Work out the finished part from the listing and answer in its coordinate system (mm). A direction names the side the tool comes from. Coordinates: 2 decimals unless noted, no trailing zeros. Loops run counter-clockwise (first coordinate to the right, second up) from the corner with the lowest first, then second, coordinate; pieces in that order, holes last. Notation, with made-up numbers: M 55,46.5 L 82,46.5 A14 cw 82,58.5 Z; hole C 6,34 d3. An arc over 180 degrees is marked long. Write each question's results on one line, items separated by ' | '.
```python
from build123d import *

# Parameters (mm, degrees)
F0_R     = 4.2
F0_W     = 2
F0_H     = 4.4
F0_W_2   = 1
F1_DEPTH = 16.4
F2_DEPTH = 6.2
F3_DEPTH = 14
F4_R     = 0.5


with BuildPart() as f1:
    # F0 (on Top) → F1 (new body)
    with BuildSketch(Plane.XY):
        Circle(F0_R)
        Polygon((-2.5, -2.2), (-2.5, 2.2), (-0.5, 2.2), (0.5, 2.2), (2.5, 2.2), (2.5, -2.2), (0.5, -2.2), (-0.5, -2.2), align=None, mode=Mode.SUBTRACT)
        with Locations((-1.5, 0)):
            Rectangle(F0_W, F0_H)
        with Locations((1.5, 0)):
            Rectangle(F0_W, F0_H)
        Rectangle(F0_W_2, F0_H)
    extrude(amount=F1_DEPTH)

    # F0 (on Top) → F2 (cut)
    with BuildSketch(Plane.XY):
        with Locations((1.5, 0)):
            Rectangle(F0_W, F0_H)
        with Locations((-1.5, 0)):
            Rectangle(F0_W, F0_H)
        Rectangle(F0_W_2, F0_H)
    extrude(amount=F2_DEPTH, mode=Mode.SUBTRACT)

    # F0 (on Top) → F3 (cut)
    with BuildSketch(Plane.XY):
        with Locations((1.5, 0)):
            Rectangle(F0_W, F0_H)
        with Locations((-1.5, 0)):
            Rectangle(F0_W, F0_H)
    extrude(amount=F3_DEPTH, mode=Mode.SUBTRACT)

    # F4
    f4_edges = [f1.edges().sort_by_distance(p)[0] for p in [
        (-4.2, 0, 16.4),
    ]]
    fillet(f4_edges, radius=F4_R)


solid = f1.part
```
1) Find section D-D, the plane x = 0. Give the vertices of the cut face in (y, z).
Check result:
outline: M -4.2,0 L -2.2,0 L -2.2,6.2 L 2.2,6.2 L 2.2,0 L 4.2,0 L 4.2,15.9 A0.5 ccw 3.7,16.4 L -3.7,16.4 A0.5 ccw -4.2,15.9 Z
2) Find section A-A, the plane z = 6.75. Give the vertices of the cut face in (x, y).
Check result:
outline: C 0,0 d8.4; hole M -2.5,-2.2 L -0.5,-2.2 L -0.5,2.2 L -2.5,2.2 Z; hole M 0.5,-2.2 L 2.5,-2.2 L 2.5,2.2 L 0.5,2.2 Z
3) Straight lines are drawn through the part: probe 1 along X at (y, z) = (-2, 13.75); probe 2 along X at (y, z) = (-1, 10.25); probe 3 along X at (y, z) = (1.25, 4.75). For each, find the intervals that lie inside material, in ascending order. Write a range as [from, to].
Check result:
probe 1: [-3.69, -2.5], [-0.5, 0.5], [2.5, 3.69] | probe 2: [-4.08, -2.5], [-0.5, 0.5], [2.5, 4.08] | probe 3: [-4.01, -2.5], [2.5, 4.01]
4) Given pin 1 Ø2 at (x, y) = (2, 0.5) entering from -Z; pin 2 Ø1.5 at (x, z) = (-3, 9.5) entering from -Y; pin 3 Ø3 at (x, z) = (2.5, 9.5) entering from -Y; pin 4 Ø1.5 at (y, z) = (2.5, 12) entering from -X, each flat-ended and moving along its own axis, determine where each tip first touches the part or whether it passes through.
Check result:
pin 1: z = 0 | pin 2: y = -3.55 | pin 3: y = -4.08 | pin 4: x = -3.82
5) Which of the six approach directions +Z, -Z, +X, -X, +Y, -Y give full straight-line access (tool end or side, diameter ignored) to faces 1 (the face through (2.5, 0, 7)), 2 (the face through (3, 0, 0))?
Check result:
face 1: -Z | face 2: -Z, +X, -X, +Y, -Y
6) Find section B-B, the plane z = 4.5. Give the vertices of the cut face in (x, y).
Check result:
outline: C 0,0 d8.4; hole M -2.5,-2.2 L 2.5,-2.2 L 2.5,2.2 L -2.5,2.2 Z
7) Find section C-C, the plane y = 0. Give the vertices of the cut face in (x, z).
Check result:
outline: M -4.2,0 L -2.5,0 L -2.5,14 L -0.5,14 L -0.5,6.2 L 0.5,6.2 L 0.5,14 L 2.5,14 L 2.5,0 L 4.2,0 L 4.2,15.9 A0.5 ccw 3.7,16.4 L -3.7,16.4 A0.5 ccw -4.2,15.9 Z
